The listing builds one solid part. Answer for the finished solid, in the listing's coordinates (mm). Round coordinates to 2 decimals unless told otherwise and drop trailing zeros. Write each loop counter-clockwise with the first axis right and the second up, starting at its lowest first coordinate (ties: lowest second). Pieces come first, ordered by that corner, then holes. Notation, with made-up numbers: (-15.75, -8) - (14.25, -8) arc R25 cw to (14.25, 17) - close; hole circle Ø10 at (1, 74.25). An arc over 180 degrees is marked (long way). Answer in a Markdown table with one row per item.
from build123d import *

# Parameters (mm, degrees)
F0_R     = 5
F1_DEPTH = 25
F2_R     = 5.5
F3_DEPTH = 1
F8_R     = 5.5
F8_R_2   = 5.3
F9_DEPTH = 1


with BuildPart() as f1:
    # F0 (on Front) → F1 (new body)
    with BuildSketch(Plane.XZ):
        Circle(F0_R)
    extrude(amount=F1_DEPTH)

    # F2 (on face) → F3 (join)
    with BuildSketch(Plane(origin=(0, 0, 0), x_dir=(-1, 0, 0), z_dir=(0, 1, 0))):
        Circle(F2_R)
    extrude(amount=-F3_DEPTH)

    # F4 (on Right) → F5 (revolve, cut)
    with BuildSketch(Plane.YZ):
        Polygon((0, 5.5), (-1, 5.5), (0, 5), align=None)
    revolve(axis=Axis((0, -11.148525, 0), (0, 1, 0)), mode=Mode.SUBTRACT)

    # F6 (on Right) → F7 (revolve, cut)
    with BuildSketch(Plane.YZ):
        Polygon((-1, 5), (-0.3, 5), (-1, 5.3), align=None)
    revolve(axis=Axis((0, -11.529621, 0), (0, 1, 0)), mode=Mode.SUBTRACT)

    # F8 (on face) → F9 (join)
    with BuildSketch(Plane.XZ.offset(1)):
        Circle(F8_R)
        Circle(F8_R_2, mode=Mode.SUBTRACT)
    extrude(amount=F9_DEPTH)


solid = f1.part
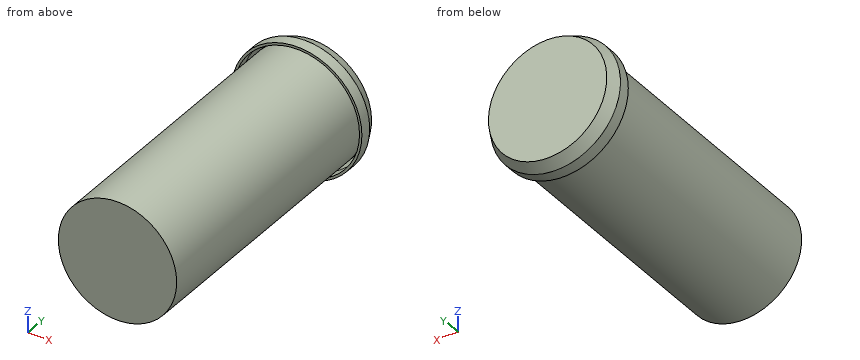
(1) Section C-C (y = -7.5) is taken. Give the vertices of the cut face in (x, z).
Checked values:
| item | result |
|---|---|
| outline | circle Ø10 at (0, 0) |
(2) Section A-A (z = 0) is taken. Give the vertices of the cut face in (x, y), and give its area (3 significant figures).
Checked values:
| item | result |
|---|---|
| outline | (-5.5, -2) - (-5.3, -2) - (-5.3, -1) - (-5, -0.3) - (-5, -25) - (5, -25) - (5, -0.3) - (5.3, -1) - (5.3, -2) - (5.5, -2) - (5.5, -1) - (5, 0) - (-5, 0) - (-5.5, -1) - close |
| area | 251 mm2 |
(3) Flat-ended cylindrical pins translate along their axes: pin 1 (5 mm diameter, centred on x = -3.5, y = -18.5, fed in from +Z); pin 2 (1.5 mm diameter, centred on y = -16.5, z = 1, fed in from +X); pin 3 (6 mm diameter, centred on y = -12, z = -4, fed in from -X). Find the tip coordinate at first contact, or state that the pin passes through.
Checked values:
| item | result |
|---|---|
| pin 1 | stops at z = 4.9 |
| pin 2 | stops at x = 4.99 |
| pin 3 | stops at x = -4.9 |
(4) Section B-B (x = 0) is taken. Give the vertices of the cut face in (y, z), and give its area (3 significant figures).
Checked values:
| item | result |
|---|---|
| outline | (-25, -5) - (-0.3, -5) - (-1, -5.3) - (-2, -5.3) - (-2, -5.5) - (-1, -5.5) - (0, -5) - (0, 5) - (-1, 5.5) - (-2, 5.5) - (-2, 5.3) - (-1, 5.3) - (-0.3, 5) - (-25, 5) - close |
| area | 251 mm2 |
(5) Find the intervals of material crossed by line 1 (X direction, y = -1.2, z = 0); line 2 (Z direction, x = -4.25, y = -1.25); line 3 (Z direction, x = -0.75, y = -18), in increasing order.
Checked values:
| item | result |
|---|---|
| line 1 | x = -5.5 to -5.3, -5 to 5, 5.3 to 5.5 |
| line 2 | z = -3.49 to -3.17, -2.63 to 2.63, 3.17 to 3.49 |
| line 3 | z = -4.94 to 4.94 |
